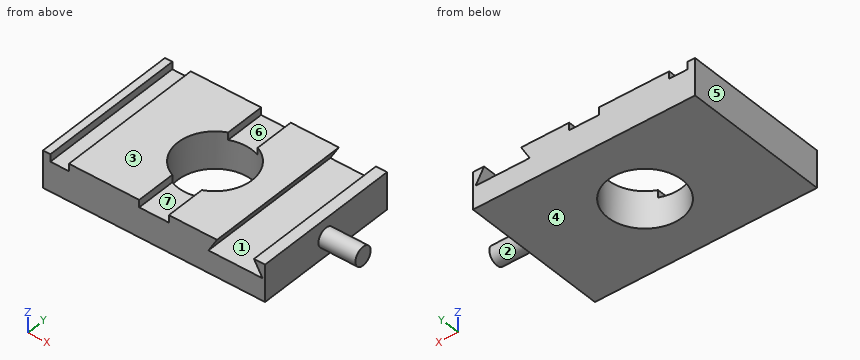
from build123d import *

# Parameters (mm, degrees)
F0_W     = 76.2
F0_H     = 50.8
F0_R     = 12.7
F1_DEPTH = 12.7
F2_W     = 6.35
F2_H     = 50.8
F3_DEPTH = 2.54
F5_DEPTH = 50.8508
F6_R     = 3.175
F7_DEPTH = 12.7


with BuildPart() as f1:
    # F0 (on Top) → F1 (new body)
    with BuildSketch(Plane.XY):
        Rectangle(F0_W, F0_H)
        Circle(F0_R, mode=Mode.SUBTRACT)
    extrude(amount=F1_DEPTH)

    # F2 (on face) → F3 (cut)
    with BuildSketch(Plane.XY.offset(12.7)):
        with BuildLine():
            ThreePointArc((5.08, -11.639742), (0, -12.7), (-5.08, -11.639742))
            Line((-5.08, -11.639742), (-5.08, -25.4))
            Line((-5.08, -25.4), (5.08, -25.4))
            Line((5.08, -25.4), (5.08, -11.639742))
        make_face()
        with BuildLine():
            Line((5.08, 25.4), (-5.08, 25.4))
            Line((-5.08, 25.4), (-5.08, 11.639742))
            ThreePointArc((-5.08, 11.639742), (0, 12.7), (5.08, 11.639742))
            Line((5.08, 11.639742), (5.08, 25.4))
        make_face()
        with Locations((-32.385, 0)):
            Rectangle(F2_W, F2_H)
    extrude(amount=-F3_DEPTH, mode=Mode.SUBTRACT)

    # F4 (on face) → F5 (cut)
    with BuildSketch(Plane.XZ.offset(25.4)):
        Polygon((34.29, 12.7), (21.59, 12.7), (18.657061, 7.62), (37.222939, 7.62), align=None)
    extrude(amount=-F5_DEPTH, mode=Mode.SUBTRACT)

    # F6 (on face) → F7 (join)
    with BuildSketch(Plane.YZ.offset(38.1)):
        with Locations((0, 6.35)):
            Circle(F6_R)
    extrude(amount=F7_DEPTH)


solid = f1.part
Part model, mm, in its own coordinate system. Face numbers are marked on the shaded views. A direction names the side the tool comes from. Round coordinates to 2 decimals unless told otherwise and drop trailing zeros. Order: outer loops, then holes, each group sorted by start corner. A loop starts at its lowest first (then second) coordinate and runs counter-clockwise, first axis right, second up. Notation, with made-up numbers: (45.25, -0.5) -> (55.25, -0.5) arc R14 cw to (55.25, 13.5) -> close; hole circle Ø3 at (57, -25.5). An arc over 180 degrees is marked (long way). Put each result on its own line as item: value.
Q1. Band-saw the part on C-C (x = 0). Give the cut face in (y, z).
From the geometry:
outline: (-25.4, 0) -> (-12.7, 0) -> (-12.7, 10.16) -> (-25.4, 10.16) -> close; (12.7, 0) -> (25.4, 0) -> (25.4, 10.16) -> (12.7, 10.16) -> close
Q2. Band-saw the part on A-A (y = 0). Give the cut face in (x, z) (3 decimals).
From the geometry:
outline: (-38.1, 0) -> (-12.7, 0) -> (-12.7, 12.7) -> (-29.21, 12.7) -> (-29.21, 10.16) -> (-35.56, 10.16) -> (-35.56, 12.7) -> (-38.1, 12.7) -> close; (12.7, 0) -> (38.1, 0) -> (38.1, 3.175) -> (50.8, 3.175) -> (50.8, 9.525) -> (38.1, 9.525) -> (38.1, 12.7) -> (34.29, 12.7) -> (37.223, 7.62) -> (18.657, 7.62) -> (21.59, 12.7) -> (12.7, 12.7) -> close
Q3. Band-saw the part on B-B (z = 6.35). Give the cut face in (x, y) (3 decimals).
From the geometry:
outline: (-38.1, -25.4) -> (38.1, -25.4) -> (38.1, -3.175) -> (50.8, -3.175) -> (50.8, 3.175) -> (38.1, 3.175) -> (38.1, 25.4) -> (-38.1, 25.4) -> close; hole circle Ø25.4 at (0, 0)
Q4. Band-saw the part on D-D (z = 11.25). Give the cut face in (x, y).
From the geometry:
outline: (-38.1, -25.4) -> (-35.56, -25.4) -> (-35.56, 25.4) -> (-38.1, 25.4) -> close; (-29.21, -25.4) -> (-5.08, -25.4) -> (-5.08, -11.64) arc R12.7 cw to (-5.08, 11.64) -> (-5.08, 25.4) -> (-29.21, 25.4) -> close; (5.08, -25.4) -> (20.75, -25.4) -> (20.75, 25.4) -> (5.08, 25.4) -> (5.08, 11.64) arc R12.7 cw to (5.08, -11.64) -> close; (35.13, -25.4) -> (38.1, -25.4) -> (38.1, 25.4) -> (35.13, 25.4) -> close
Q5. Wall check: line 1 (Y direction, x = 0, z = 3.5); line 2 (X direction, y = -7.5, z = 11); line 3 (X direction, y = 11, z = 12). Give the ranges that are in metal, low to high. Write a range as [from, to].
From the geometry:
line 1: y = [-25.4, -12.7], [12.7, 25.4]
line 2: x = [-38.1, -35.56], [-29.21, -10.25], [10.25, 20.61], [35.27, 38.1]
line 3: x = [-38.1, -35.56], [-29.21, -6.35], [6.35, 21.19], [34.69, 38.1]
Q6. Pull direction X, two halves, no side cores. Call the marked faces 4, 5, 6 and 7: pulls with the +X half, pulls with the -X half, needs draft (parallel to the pull), parting line crosses it, or undercut.
From the geometry:
face 4: needs draft
face 5: pulls with the -X half
face 6: undercut
face 7: undercut
Q7. Pin check, flat tips, straight feed: pin 1 Ø1.3 at (y, z) = (17.5, 11) entering from +X; pin 2 Ø1.9 at (x, y) = (-33.5, 9) entering from +Z; pin 3 Ø3 at (x, y) = (25, -14.5) entering from +Z. Stop position of each tip, or through.
From the geometry:
pin 1: stops at x = 38.1
pin 2: stops at z = 10.16
pin 3: stops at z = 7.62
Q8. Tool access for the marked faces 1, 2 and 3: list every direction of +Z, -Z, +X, -X, +Y, -Y with a clear straight run to the whole face (end or side of a thin tool).
From the geometry:
face 1: +Y, -Y
face 2: +X
face 3: +Z, +X, -X, +Y, -Y
